Could you check a few things on this drawing? It's one solid part, dimensions in mm from its lowest x, y, z. A direction names the side the tool comes from. Coordinates: 2 decimals unless noted, no trailing zeros. Write each loop counter-clockwise with the first axis right and the second up, starting at its lowest first coordinate (ties: lowest second). Pieces come first, ordered by that corner, then holes.
Item 1: I want a section at B-B (x = 1.5). Please give me the cut outline in (y, z).
Item 2: Please list where these lines run through material, in increasing order: line 1 (X direction, y = 3.9, z = 26); line 2 (Y direction, x = 1.5, z = 23); line 3 (X direction, y = 1.5, z = 19) (3 decimals).
Item 3: I want a section at D-D (y = 2.15). Please give me the cut outline in (x, z) (3 decimals).
Item 4: I want a section at A-A (z = 19). Please give me the cut outline in (x, y) (3 decimals), and give its area (3 significant figures).
Item 5: I'm going to push a flat-ended pin straight in: P1, Ø4, axis at x = 4.5, z = 12, coming from the -Y side. Where does the tip first touch, or does it pass through?
Item 6: I want a section at C-C (y = 3.6). Please give me the cut outline in (x, z) (3 decimals), and give its area (3 significant figures).
Item 7: For the marked faces 1 and 2, which set-ups out of +Z, -Z, +X, -X, +Y, -Y let a thin tool reach every point of the face, with its end or its side?
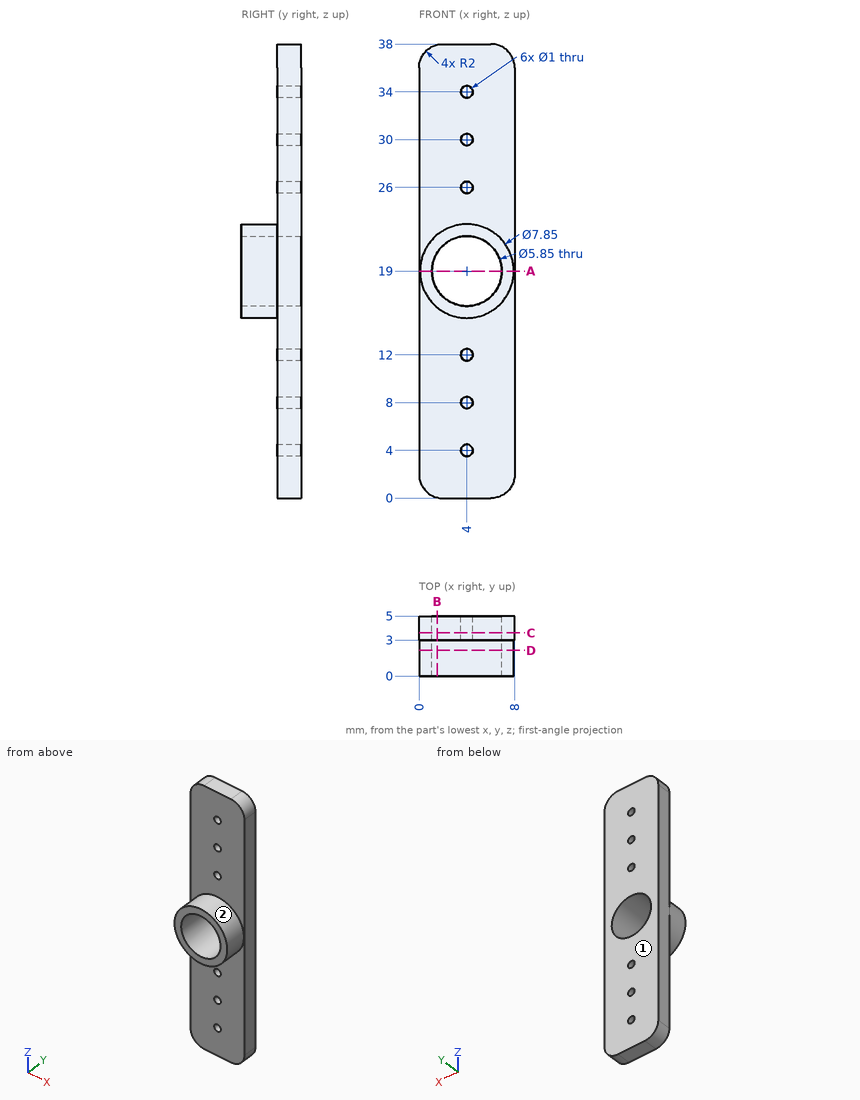
Answer:
1. outline: (0, 15.97) - (3, 15.97) - (3, 0.06) - (5, 0.06) - (5, 17.48) - (0, 17.48) - close; (0, 20.52) - (5, 20.52) - (5, 37.94) - (3, 37.94) - (3, 22.03) - (0, 22.03) - close
2. line 1: x = 0 to 3.5, 4.5 to 8
2. line 2: y = 3 to 5
2. line 3: x = 0.075 to 1.075, 6.925 to 7.925
3. outline: circle Ø7.85 at (4, 19); hole circle Ø5.85 at (4, 19)
4. outline: (0, 3) - (0.075, 3) - (0.075, 0) - (1.075, 0) - (1.075, 5) - (0, 5) - close; (6.925, 0) - (7.925, 0) - (7.925, 3) - (8, 3) - (8, 5) - (6.925, 5) - close
4. area: 10.3 mm2
5. P1: stops at y = 3
6. outline: (0, 2) arc R2 ccw to (2, 0) - (6, 0) arc R2 ccw to (8, 2) - (8, 36) arc R2 ccw to (6, 38) - (2, 38) arc R2 ccw to (0, 36) - close; hole circle Ø5.85 at (4, 19); hole circle Ø1 at (4, 4); hole circle Ø1 at (4, 8); hole circle Ø1 at (4, 12); hole circle Ø1 at (4, 26); hole circle Ø1 at (4, 30); hole circle Ø1 at (4, 34)
6. area: 269 mm2
7. face 1: +Z, -Z, +X, -X, +Y
7. face 2: -Y
